The model under review builds one solid part; all positions refer to its coordinate system, in mm. Round coordinates to 2 decimals unless told otherwise and drop trailing zeros. Write each loop counter-clockwise with the first axis right and the second up, starting at its lowest first coordinate (ties: lowest second). Pieces come first, ordered by that corner, then holes.
Item 1: Add section B-B (z = 0). Give the boundary of the cut face in (x, y), plus the area to 3 significant figures.
Item 2: Add section D-D (z = 23.5). Give the boundary of the cut face in (x, y).
Item 3: To check wall thickness, follow L1, parallel to Y at x = -7.5, z = 18.5; L2, parallel to Y at x = 11.2, z = 0; L3, parallel to Y at x = 4.5, z = 6. State the ranges of each line that lie inside material, in increasing order.
Item 4: Add section A-A (y = 0). Give the boundary of the cut face in (x, z), plus the area to 3 significant figures.
Item 5: Clearance check with flat-ended pins moving along their axes: pin 1 Ø3.5 at (y, z) = (-8.5, -15.5) entering from +X; pin 2 Ø4 at (x, y) = (-7.5, 15) entering from -Z; pin 3 Ø3 at (x, y) = (-7.5, -15) entering from -Z. State where each tip first meets the part, or that it passes through.
Item 6: Add section C-C (x = 3.75). Give the boundary of the cut face in (y, z), plus the area to 3 significant figures.
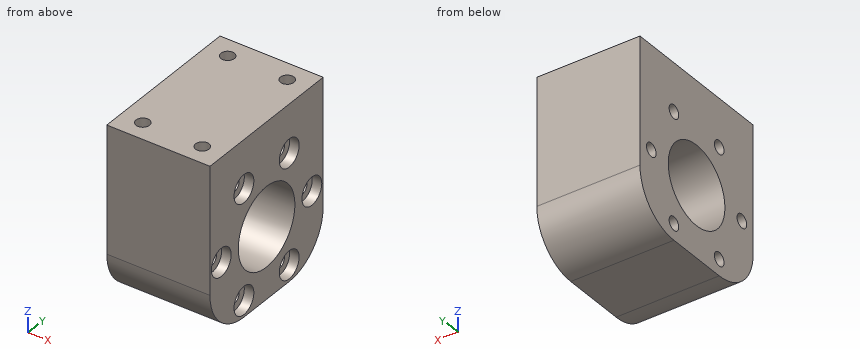
```python
from build123d import *

# Parameters (mm, degrees)
CROQUIS1_W                                           = 26
CROQUIS1_H                                           = 40
SALIENTE_EXTRUIR1_DEPTH                              = 26
TALADRO_DE_MARGEN_PARA_M31_D                         = 3.4
TALADRO_DE_MARGEN_PARA_M31_DEPTH                     = 15
TALADRO_DE_MARGEN_PARA_M31_TIP                       = 1.021463052
REFRENTADO_PARA_TORNILLO_CON_CABEZA_TRON_D           = 3.4
REFRENTADO_PARA_TORNILLO_CON_CABEZA_TRON_CBORE_D     = 7
REFRENTADO_PARA_TORNILLO_CON_CABEZA_TRON_CBORE_DEPTH = 2.4
CROQUIS7_R                                           = 10
CORTAR_EXTRUIR1_DEPTH                                = 42.856899073
CROQUIS9_W                                           = 8
CROQUIS9_H                                           = 40
CORTAR_EXTRUIR3_DEPTH                                = 42.856899073
REDONDEO3_R                                          = 12


with BuildPart() as part:
    # Croquis1 → Saliente-Extruir1 (new, symmetric)
    with BuildSketch(Plane.XY):
        Rectangle(CROQUIS1_W, CROQUIS1_H)
    extrude(amount=SALIENTE_EXTRUIR1_DEPTH, both=True)

    # Taladro de margen para M31
    with Locations(Plane.XY.offset(26)):
        with Locations((-7.5, 15), (7.5, -15), (7.5, 15), (-7.5, -15)):
            Hole(TALADRO_DE_MARGEN_PARA_M31_D / 2, depth=TALADRO_DE_MARGEN_PARA_M31_DEPTH)
            with Locations((0, 0, -(TALADRO_DE_MARGEN_PARA_M31_DEPTH + TALADRO_DE_MARGEN_PARA_M31_TIP / 2))):  # 118° drill point
                Cone(0, TALADRO_DE_MARGEN_PARA_M31_D / 2, TALADRO_DE_MARGEN_PARA_M31_TIP, mode=Mode.SUBTRACT)

    # Refrentado para tornillo con cabeza troncocónica de M31 (through all)
    with Locations(Plane(origin=(13, 0, 0), x_dir=(0, 0, -1), z_dir=(1, 0, 0))):
        with Locations((0, 16), (13.856406461, 8), (13.856406461, -8), (0, -16), (-13.856406461, -8), (-13.856406461, 8)):
            CounterBoreHole(REFRENTADO_PARA_TORNILLO_CON_CABEZA_TRON_D / 2, REFRENTADO_PARA_TORNILLO_CON_CABEZA_TRON_CBORE_D / 2, REFRENTADO_PARA_TORNILLO_CON_CABEZA_TRON_CBORE_DEPTH)

    # Croquis7 → Cortar-Extruir1 (cut, through all)
    with BuildSketch(Plane.ZY.offset(13)):
        Circle(CROQUIS7_R)
    extrude(amount=-CORTAR_EXTRUIR1_DEPTH, mode=Mode.SUBTRACT)

    # Croquis9 → Cortar-Extruir3 (cut, through all)
    with BuildSketch(Plane(origin=(13, 0, 0), x_dir=(0, 0, -1), z_dir=(1, 0, 0))):
        with Locations((22, 0)):
            Rectangle(CROQUIS9_W, CROQUIS9_H)
    extrude(amount=-CORTAR_EXTRUIR3_DEPTH, mode=Mode.SUBTRACT)

    # Redondeo3
    redondeo3_edges = [part.edges().sort_by_distance(p)[0] for p in [
        (0, -20, -18),
        (0, 20, -18),
    ]]
    fillet(redondeo3_edges, radius=REDONDEO3_R)


solid = part.part
```
Numbers:
1. outline: (-13, -20) - (13, -20) - (13, -19.5) - (10.6, -19.5) - (10.6, -17.7) - (-13, -17.7) - close; (-13, -14.3) - (10.6, -14.3) - (10.6, -12.5) - (13, -12.5) - (13, -10) - (-13, -10) - close; (-13, 10) - (13, 10) - (13, 12.5) - (10.6, 12.5) - (10.6, 14.3) - (-13, 14.3) - close; (-13, 17.7) - (10.6, 17.7) - (10.6, 19.5) - (13, 19.5) - (13, 20) - (-13, 20) - close
1. area: 326 mm2
2. outline: (-13, -20) - (13, -20) - (13, 20) - (-13, 20) - close; hole circle Ø3.4 at (-7.5, -15); hole circle Ø3.4 at (-7.5, 15); hole circle Ø3.4 at (7.5, -15); hole circle Ø3.4 at (7.5, 15)
3. L1: y = -20 to -16.7, -13.3 to 13.3, 16.7 to 20
3. L2: y = -20 to -19.5, -12.5 to -10, 10 to 12.5, 19.5 to 20
3. L3: y = -20 to -8, 8 to 20
4. outline: (-13, -18) - (13, -18) - (13, -10) - (-13, -10) - close; (-13, 10) - (13, 10) - (13, 26) - (-13, 26) - close
4. area: 624 mm2
5. pin 1: stops at x = 10.6
5. pin 2: stops at z = -16.91
5. pin 3: stops at z = -16.67
6. outline: (-20, -6) arc R12 ccw to (-8, -18) - (8, -18) arc R12 ccw to (20, -6) - (20, 26) - (-20, 26) - close; hole circle Ø3.4 at (-16, 0); hole circle Ø20 at (0, 0); hole circle Ø3.4 at (-8, -13.86); hole circle Ø3.4 at (-8, 13.86); hole circle Ø3.4 at (8, -13.86); hole circle Ø3.4 at (8, 13.86); hole circle Ø3.4 at (16, 0)
6. area: 1,330 mm2
